```python
from build123d import *

# Parameters (mm, degrees)
EXTRUDE_1_DEPTH = 1


with BuildPart() as part:
    # 草圖1 → 填料-伸長1 (new body)
    with BuildSketch(Plane(origin=(0, 0, 0), x_dir=(1, 0, 0), z_dir=(0, 1, 0))):
        with BuildLine():
            Line((0, 0), (76, 0))
            Line((76, 0), (76, 2))
            Line((76, 2), (81, 2))
            Line((81, 2), (81, 6))
            Line((81, 6), (77, 6))
            Line((77, 6), (77, 7.5))
            Line((77, 7.5), (81, 7.5))
            Line((81, 7.5), (81, 18.5))
            Line((81, 18.5), (77, 18.5))
            Line((77, 18.5), (77, 20))
            Line((77, 20), (81, 20))
            Line((81, 20), (81, 24))
            Line((81, 24), (76, 24))
            Line((76, 24), (76, 26))
            Line((76, 26), (0, 26))
            Line((0, 26), (0, 15))
            ThreePointArc((0, 15), (2, 13), (0, 11))
            Line((0, 11), (0, 0))
        make_face()
    extrude(amount=EXTRUDE_1_DEPTH)


solid = part.part
```
Work out the finished part from the listing and answer in its coordinate system (mm). Give positions to 0.01 mm unless a question says otherwise; leave off trailing zeros. Loops run counter-clockwise (first coordinate to the right, second up) from the corner with the lowest first, then second, coordinate; pieces in that order, holes last. Notation, with made-up numbers: (67, 9) -> (125, 9) arc R16 ccw to (125, 35) -> close; hole circle Ø11 at (70, 0.25). An arc over 180 degrees is marked (long way). Use CSV: the item, a comma, the result in double quotes.
1. The part is cut by section A-A (y = 0.3). Write down the section's boundary in (x, z), then the cut area to 3 significant figures.
Found:
outline,"(0, -26) -> (76, -26) -> (76, -24) -> (81, -24) -> (81, -20) -> (77, -20) -> (77, -18.5) -> (81, -18.5) -> (81, -7.5) -> (77, -7.5) -> (77, -6) -> (81, -6) -> (81, -2) -> (76, -2) -> (76, 0) -> (0, 0) -> (0, -11) arc R2 cw to (0, -15) -> close"
area,"2,070 mm^2"
2. The part is cut by section B-B (z = -13). Write down the section's boundary in (x, y).
Found:
outline,"(2, 0) -> (81, 0) -> (81, 1) -> (2, 1) -> close"
3. Straight lines are drawn through the part: line 1 (X direction, y = 0.5, z = -1.5); line 2 (X direction, y = 0.15, z = -19.75). For each, find the intervals that lie inside material, in ascending order.
Found:
line 1,"0 to 76"
line 2,"0 to 77"
4. Flat-ended cylindrical pins translate along their axes: pin 1 Ø0.5 at (x, y) = (80, 0.5) entering from -Z; pin 2 Ø0.5 at (x, y) = (77.5, 0.5) entering from +Z. Find the tip coordinate at first contact, or state that the pin passes through.
Found:
pin 1,"z = -24"
pin 2,"z = -2"
